from build123d import *

# Parameters (mm, degrees)
SALIENTE_EXTRUIR1_DEPTH = 3
CROQUIS2_W              = 3
CROQUIS2_H              = 15
SALIENTE_EXTRUIR2_DEPTH = 3
CROQUIS3_W              = 2.5
CROQUIS3_H              = 15
SALIENTE_EXTRUIR3_DEPTH = 17
CROQUIS4_W              = 15.5
CROQUIS4_H              = 3
SALIENTE_EXTRUIR4_DEPTH = 68
CROQUIS5_W              = 15.5
CROQUIS5_H              = 5
SALIENTE_EXTRUIR5_DEPTH = 10
CROQUIS6_W              = 15.5
CROQUIS6_H              = 5
SALIENTE_EXTRUIR6_DEPTH = 10
CORTAR_EXTRUIR1_DEPTH   = 10
CORTAR_EXTRUIR2_DEPTH   = 10
REDONDEO2_R             = 0.5


with BuildPart() as part:
    # Croquis1 → Saliente-Extruir1 (new body)
    with BuildSketch(Plane(origin=(0, 0, 0), x_dir=(1, 0, 0), z_dir=(0, 1, 0))):
        Polygon((-28.106357332, -8.17639486), (11.393642668, -8.17639486), (11.393642668, -24.07639486), (26.893642668, -24.07639486), (26.893642668, -7.17639486), (26.893642668, 7.82360514), (-12.606357332, 7.82360514), (-12.606357332, 23.72360514), (-28.106357332, 23.72360514), (-28.106357332, 6.82360514), align=None)
    extrude(amount=SALIENTE_EXTRUIR1_DEPTH)

    # Croquis2 → Saliente-Extruir2 (add)
    with BuildSketch(Plane(origin=(0, 3, 0), x_dir=(1, 0, 0), z_dir=(0, 1, 0))):
        with Locations((28.393642668, 0.32360514)):
            Rectangle(CROQUIS2_W, CROQUIS2_H)
        with Locations((-29.606357332, -0.67639486)):
            Rectangle(CROQUIS2_W, CROQUIS2_H)
    extrude(amount=-SALIENTE_EXTRUIR2_DEPTH)

    # Croquis3 → Saliente-Extruir3 (add)
    with BuildSketch(Plane.XZ):
        with Locations((-29.856357332, 0.67639486)):
            Rectangle(CROQUIS3_W, CROQUIS3_H)
        with Locations((28.643642668, -0.32360514)):
            Rectangle(CROQUIS3_W, CROQUIS3_H)
    extrude(amount=SALIENTE_EXTRUIR3_DEPTH)

    # Croquis4 → Saliente-Extruir4 (add)
    with BuildSketch(Plane.XZ):
        with Locations((-20.356357332, -22.22360514)):
            Rectangle(CROQUIS4_W, CROQUIS4_H)
        with Locations((19.143642668, 22.57639486)):
            Rectangle(CROQUIS4_W, CROQUIS4_H)
    extrude(amount=SALIENTE_EXTRUIR4_DEPTH)

    # Croquis5 → Saliente-Extruir5 (add)
    with BuildSketch(Plane(origin=(0, 0, -23.72360514), x_dir=(-1, 0, 0), z_dir=(0, 0, -1))):
        with Locations((20.356357332, -65.5)):
            Rectangle(CROQUIS5_W, CROQUIS5_H)
    extrude(amount=SALIENTE_EXTRUIR5_DEPTH)

    # Croquis6 → Saliente-Extruir6 (add)
    with BuildSketch(Plane.XY.offset(24.07639486)):
        with Locations((19.143642668, -65.5)):
            Rectangle(CROQUIS6_W, CROQUIS6_H)
    extrude(amount=SALIENTE_EXTRUIR6_DEPTH)

    # Croquis7 → Cortar-Extruir1 (cut)
    with BuildSketch(Plane(origin=(0, -63, 0), x_dir=(1, 0, 0), z_dir=(0, 1, 0))):
        with BuildLine():
            Line((16.043642668, -29.07639486), (16.043642668, -34.07639486))
            Line((16.043642668, -34.07639486), (22.243642668, -34.07639486))
            Line((22.243642668, -34.07639486), (22.243642668, -29.07639486))
            ThreePointArc((22.243642668, -29.07639486), (19.143642668, -25.97639486), (16.043642668, -29.07639486))
        make_face()
    extrude(amount=-CORTAR_EXTRUIR1_DEPTH, mode=Mode.SUBTRACT)

    # Croquis8 → Cortar-Extruir2 (cut)
    with BuildSketch(Plane(origin=(0, -63, 0), x_dir=(1, 0, 0), z_dir=(0, 1, 0))):
        with BuildLine():
            Line((-23.456357332, 28.72360514), (-23.456357332, 33.72360514))
            Line((-23.456357332, 33.72360514), (-17.256357332, 33.72360514))
            Line((-17.256357332, 33.72360514), (-17.256357332, 28.72360514))
            ThreePointArc((-17.256357332, 28.72360514), (-20.356357332, 25.62360514), (-23.456357332, 28.72360514))
        make_face()
    extrude(amount=-CORTAR_EXTRUIR2_DEPTH, mode=Mode.SUBTRACT)

    # Redondeo2
    redondeo2_edges = [part.edges().sort_by_distance(p)[0] for p in [
        (19.143642668, -63, 24.07639486),
        (19.143642668, 0, 21.07639486),
        (27.393642668, 0, -0.32360514),
        (-28.606357332, 0, 0.67639486),
        (-20.356357332, 0, -20.72360514),
        (-20.356357332, -63, -23.72360514),
    ]]
    fillet(redondeo2_edges, radius=REDONDEO2_R)


solid = part.part
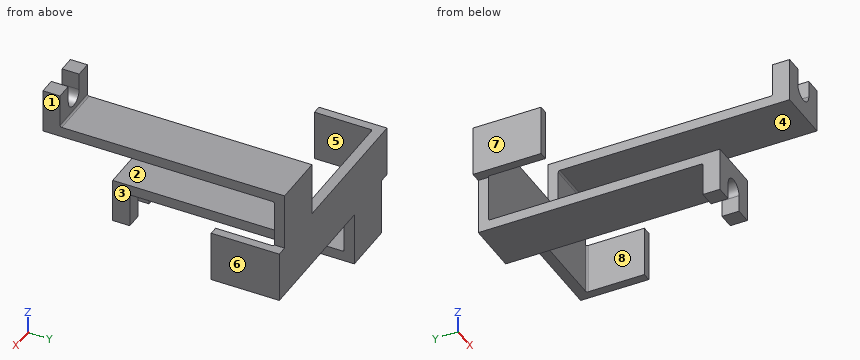
Geometry: final body of the model. Coordinates: model frame, mm. Face numbers are marked on the shaded views. A direction names the side the tool comes from. Give positions to 0.01 mm unless a question says otherwise; leave off trailing zeros. Order: outer loops, then holes, each group sorted by start corner. A loop starts at its lowest first (then second) coordinate and runs counter-clockwise, first axis right, second up. Notation, with made-up numbers: (13.25, 44.5) -> (72.25, 44.5) arc R24 cw to (72.25, 62.5) -> close; hole circle Ø5 at (75, 17). An arc over 180 degrees is marked (long way). Put each result on its own line as item: value.
Q1. Material intervals for L1, parallel to X at y = -5.5, z = -6.5; L2, parallel to Z at x = -26.5, y = -26; L3, parallel to Z at x = 13, y = -25.5, sorted ascending.
Here are the results:
L1: x = -31.11 to -28.61, 27.39 to 29.89
L2: z = -23.72 to -20.72
L3: z = 21.08 to 24.08
Q2. Section D-D, the plane x = 13. Return loops of the section in (y, z), then the cut area to 3 significant figures.
Here are the results:
outline: (-68, 21.08) -> (-0.5, 21.08) arc R0.5 cw to (0, 20.58) -> (0, -7.82) -> (3, -7.82) -> (3, 24.08) -> (-62.5, 24.08) arc R0.5 cw to (-63, 24.58) -> (-63, 34.08) -> (-68, 34.08) -> close
area: 350 mm^2
Q3. Draft query along X for the marked faces 5, 6, 7 and 8. Return one class per face: released by +X, released by -X, zero draft, split by the parting line, or undercut.
Here are the results:
face 5: undercut
face 6: released by +X
face 7: released by -X
face 8: undercut
Q4. Section A-A, the plane y = -43.5. Return loops of the section in (x, z), then the cut area to 3 significant figures.
Here are the results:
outline: (-28.11, -23.72) -> (-12.61, -23.72) -> (-12.61, -20.72) -> (-28.11, -20.72) -> close; (11.39, 21.08) -> (26.89, 21.08) -> (26.89, 24.08) -> (11.39, 24.08) -> close
area: 93.0 mm^2
Q5. Section B-B, the plane y = -15. Return loops of the section in (x, z), then the cut area to 3 significant figures.
Here are the results:
outline: (-31.11, -6.82) -> (-28.61, -6.82) -> (-28.61, 8.18) -> (-31.11, 8.18) -> close; (-28.11, -23.72) -> (-12.61, -23.72) -> (-12.61, -20.72) -> (-28.11, -20.72) -> close; (11.39, 21.08) -> (26.89, 21.08) -> (26.89, 24.08) -> (11.39, 24.08) -> close; (27.39, -7.82) -> (29.89, -7.82) -> (29.89, 7.18) -> (27.39, 7.18) -> close
area: 168 mm^2
Q6. Section C-C, the plane z = 3.5. Return loops of the section in (x, y).
Here are the results:
outline: (-31.11, -17) -> (-28.61, -17) -> (-28.61, -0.5) arc R0.5 cw to (-28.11, 0) -> (26.89, 0) arc R0.5 cw to (27.39, -0.5) -> (27.39, -17) -> (29.89, -17) -> (29.89, 3) -> (-31.11, 3) -> close
Q7. Pin query (flat end, axial travel): pin 1 (3 mm diameter, centred on x = -11.5, y = -4.5, fed in from +Z); pin 2 (4 mm diameter, centred on x = -14, y = -23, fed in from -Z); pin 3 (12.5 mm diameter, centred on x = 19.5, y = -19, fed in from +Z). Return the tip coordinate at first contact, or that it passes through.
Here are the results:
pin 1: stops at z = -20.72
pin 2: stops at z = -23.72
pin 3: stops at z = 24.08
Q8. Reachability of the marked faces 1, 2, 3 and 4 from +Z, -Z, +X, -X, +Y, -Y: full face, straight path, thin tool, end or side. Return the list, or none.
Here are the results:
face 1: +Z, +X, +Y, -Y
face 2: +Z, +X, -X, -Y
face 3: -Z, +X, +Y, -Y
face 4: -Z, +X, -X, -Y
